from build123d import *

# Parameters (mm, degrees)
SKETCH1_W           = 25.4
SKETCH1_H           = 25.4
BOSS_EXTRUDE1_DEPTH = 5.588
BOSS_EXTRUDE2_DEPTH = 38.1


with BuildPart() as part:
    # Sketch1 → Boss-Extrude1 (new body)
    with BuildSketch(Plane(origin=(0, 0, 0), x_dir=(1, 0, 0), z_dir=(0, 1, 0))):
        Rectangle(SKETCH1_W, SKETCH1_H)
    extrude(amount=BOSS_EXTRUDE1_DEPTH)

    # Sketch2 → Boss-Extrude2 (add)
    with BuildSketch(Plane(origin=(0, 5.588, 0), x_dir=(1, 0, 0), z_dir=(0, 1, 0))):
        Polygon((-7.004599774, 10.955912468), (10.955912468, -7.004599774), (7.004599774, -10.955912468), (-10.955912468, 7.004599774), align=None)
    extrude(amount=BOSS_EXTRUDE2_DEPTH)


solid = part.part
Source: CAD feature listing. Evaluate the final solid. Frame: model axes, mm. A direction names the side the tool comes from. Round coordinates to 2 decimals unless told otherwise and drop trailing zeros. Write each loop counter-clockwise with the first axis right and the second up, starting at its lowest first coordinate (ties: lowest second). Pieces come first, ordered by that corner, then holes. Notation, with made-up numbers: (-10.5, 34.5) - (41.5, 34.5) arc R10 ccw to (41.5, 48.5) - close; hole circle Ø6 at (-33, 26). An arc over 180 degrees is marked (long way). Use CSV: the item, a comma, the result in double quotes. Start each with the question number.
(1) Cut plane B-B, the plane x = -4.5. Return loops of the section in (y, z), and give its area (3 significant figures).
(2) Set-up query: faces 1 (the face through (3, 5.588, -3)), 2 (the face through (1.85, 24.37, -2.1)), 3 (the face through (-9.01, 24.37, -8.95)), 4 (the face through (9.01, 24.37, 8.95)). Return all of +Z, -Z, +X, -X, +Y, -Y with unobstructed straight access to the full face (end or side cutting, diameter ignored); none if empty.
(3) First-contact query: pin 1 Ø5 at (x, y) = (8.5, 38) entering from +Z; pin 2 Ø1 at (y, z) = (38, -8) entering from +X; pin 3 Ø5 at (x, y) = (0.5, 12.5) entering from -Z. Flat tips, straight axial feed; report the tip coordinate or a pass-through.
(4) Cut plane C-C, the plane y = 31. Return loops of the section in (x, z), and give its area (3 significant figures).
(5) Material intervals for probe 1 along Y at (x, z) = (1.25, 11.75); probe 2 along X at (y, z) = (33.5, 2); probe 3 along Z at (x, y) = (-10.75, 26.5), sorted ascending. Write a range as [from, to].
(6) Cut plane A-A, the plane z = -8.75. Return loops of the section in (x, y), and give its area (3 significant figures).
Geometry says:
1,outline,"(0, -12.7) - (5.59, -12.7) - (5.59, -8.45) - (43.69, -8.45) - (43.69, -0.55) - (5.59, -0.55) - (5.59, 12.7) - (0, 12.7) - close"
1,area,"443 mm²"
2,face 1,"+Y"
2,face 2,"-Z, +X, +Y"
2,face 3,"-Z, -X, +Y"
2,face 4,"+Z, +X, +Y"
3,pin 1,"z = 10.96"
3,pin 2,"x = -3.55"
3,pin 3,"z = -5.95"
4,outline,"(-10.96, -7) - (-7, -10.96) - (10.96, 7) - (7, 10.96) - close"
4,area,"142 mm²"
5,probe 1,"[0, 5.59]"
5,probe 2,"[-1.95, 5.95]"
5,probe 3,"[-7.21, -6.8]"
6,outline,"(-12.7, 0) - (12.7, 0) - (12.7, 5.59) - (-4.8, 5.59) - (-4.8, 43.69) - (-9.21, 43.69) - (-9.21, 5.59) - (-12.7, 5.59) - close"
6,area,"310 mm²"
